from build123d import *

# Parameters (mm, degrees)
BOSS_EXTRUDE1_DEPTH   = 7.62
BOSS_EXTRUDE1_2_DEPTH = 7.62
BOSS_EXTRUDE1_3_DEPTH = 7.62
BOSS_EXTRUDE1_4_DEPTH = 7.62
SKETCH2_W             = 132.9538108
SKETCH2_H             = 20
BOSS_EXTRUDE2_DEPTH   = 6.35
LPATTERN2_COUNT       = 2
LPATTERN2_PITCH       = 75.4126
CUT_EXTRUDE1_DEPTH    = 125.148300392
FILLET1_R             = 2.54
SKETCH6_W             = 25.4
SKETCH6_H             = 25.4
BOSS_EXTRUDE7_DEPTH   = 12.7
FILLET3_R             = 7.62
FILLET5_R             = 7.62
SKETCH11_R            = 1.984375
CUT_EXTRUDE3_DEPTH    = 137.653262418
SKETCH13_R            = 3.5
CUT_EXTRUDE5_DEPTH    = 127.945019246
FILLET6_R             = 2.54


with BuildPart() as part:
    # Sketch1 → Boss-Extrude1 (new body)
    with BuildSketch(Plane(origin=(0, 0, 0), x_dir=(1, 0, 0), z_dir=(0, 1, 0))):
        Polygon((-2.9718, 10), (-2.9718, 7.714), (-4.4450054, 7.714), (-4.4450054, 6.444), (-2.9718, 4.158), (2.9718, 4.158), (4.4449946, 6.444), (4.4449946, 7.714), (2.9718, 7.714), (2.9718, 10), align=None)
    boss_extrude1 = extrude(amount=BOSS_EXTRUDE1_DEPTH)



with BuildPart() as body_2:
    # Sketch1 → Boss-Extrude1 2 (new body)
    with BuildSketch(Plane(origin=(0, 0, 0), x_dir=(1, 0, 0), z_dir=(0, 1, 0))):
        Polygon((4.158, -2.9718), (4.158, 2.9718), (6.444, 4.4449946), (7.714, 4.4449946), (7.714, 2.9718), (10, 2.9718), (10, -2.9718), (7.714, -2.9718), (7.714, -4.4450054), (6.444, -4.4450054), align=None)
    boss_extrude1_2 = extrude(amount=BOSS_EXTRUDE1_2_DEPTH)


with BuildPart() as body_3:
    # Sketch1 → Boss-Extrude1 3 (new body)
    with BuildSketch(Plane(origin=(0, 0, 0), x_dir=(1, 0, 0), z_dir=(0, 1, 0))):
        Polygon((4.4450054, -6.444), (2.9718, -4.158), (-2.9718, -4.158), (-4.4449946, -6.444), (-4.4449946, -7.714), (-2.9718, -7.714), (-2.9718, -10), (2.9718, -10), (2.9718, -7.714), (4.4450054, -7.714), align=None)
    boss_extrude1_3 = extrude(amount=BOSS_EXTRUDE1_3_DEPTH)


with BuildPart() as body_4:
    # Sketch1 → Boss-Extrude1 4 (new body)
    with BuildSketch(Plane(origin=(0, 0, 0), x_dir=(1, 0, 0), z_dir=(0, 1, 0))):
        Polygon((-10, -2.9718), (-10, 2.9718), (-7.714, 2.9718), (-7.714, 4.4450054), (-6.444, 4.4450054), (-4.158, 2.9718), (-4.158, -2.9718), (-6.444, -4.4449946), (-7.714, -4.4449946), (-7.714, -2.9718), align=None)
    boss_extrude1_4 = extrude(amount=BOSS_EXTRUDE1_4_DEPTH)


with BuildPart() as part_1:
    add(part.part)

    add(body_2.part)  # Boss-Extrude2 merges body 2

    add(body_3.part)  # Boss-Extrude2 merges body 3

    add(body_4.part)  # Boss-Extrude2 merges body 4
    # Sketch2 → Boss-Extrude2 (add)
    with BuildSketch(Plane.XZ):
        with Locations((-56.4769054, 0)):
            Rectangle(SKETCH2_W, SKETCH2_H)
    extrude(amount=BOSS_EXTRUDE2_DEPTH)

    # LPattern2: Boss-Extrude1, Boss-Extrude1 2, Boss-Extrude1 3, Boss-Extrude1 4 ×2
    with Locations(*[(-i * LPATTERN2_PITCH, 0, 0) for i in range(1, LPATTERN2_COUNT)]):
        add(boss_extrude1)
        add(boss_extrude1_2)
        add(boss_extrude1_3)
        add(boss_extrude1_4)

    # Sketch4 → Cut-Extrude1 (cut, through all)
    with BuildSketch(Plane(origin=(0, -6.35, 0), x_dir=(-1, 0, 0), z_dir=(0, -1, 0))):
        Polygon((122.9538108, -10), (85.4126108, -10), (122.9538108, -0.2108), align=None)
    extrude(amount=-CUT_EXTRUDE1_DEPTH, mode=Mode.SUBTRACT)

    # Fillet1
    fillet1_edges = [part_1.edges().sort_by_distance(p)[0] for p in [
        (-85.4126108, -3.175, 10),
    ]]
    fillet(fillet1_edges, radius=FILLET1_R)

    # Sketch6 → Boss-Extrude7 (add)
    with BuildSketch(Plane.ZY.offset(122.9538108)):
        with Locations((-12.4892, 6.35)):
            Rectangle(SKETCH6_W, SKETCH6_H)
    extrude(amount=-BOSS_EXTRUDE7_DEPTH)

    # Fillet3
    fillet3_edges = [part_1.edges().sort_by_distance(p)[0] for p in [
        (-110.2538108, 0, -4.8946),
        (-110.2538108, -3.175, -10),
    ]]
    fillet(fillet3_edges, radius=FILLET3_R)

    # Fillet5
    # the kernel refuses this fillet: 7.62 mm, written as the material it takes off along each edge
    with BuildSketch(Plane(origin=(-110.2538108, 38.1, 0.2108), x_dir=(-1, 0, 0), z_dir=(0, -1, 0))) as fillet5_piece_1:
        with BuildLine():
            CenterArc((FILLET5_R, FILLET5_R), FILLET5_R, 180, 90)
            Line((0, FILLET5_R), (0, 0))
            Line((0, 0), (FILLET5_R, 0))
        make_face()
    extrude(amount=30.48, mode=Mode.SUBTRACT)
    with BuildSketch(Plane(origin=(-102.6338108, 7.62, 0.2108), x_dir=(0.5976672776328267, 0.8017442392976488, 0), z_dir=(-0.8017442392976488, 0.5976672776328267, 0))) as fillet5_piece_2_section:
        with BuildLine():
            CenterArc((7.62 + FILLET5_R, FILLET5_R), FILLET5_R, 180, 90)
            Line((7.62, FILLET5_R), (7.62, 0))
            Line((7.62, 0), (7.62 + FILLET5_R, 0))
        make_face()
    fillet5_piece_2 = revolve(axis=Axis((-102.6338108, 7.62, 0.2108), (0, 0, -1)), revolution_arc=233.296989237, mode=Mode.PRIVATE)
    fillet5_piece_2 = split(fillet5_piece_2, bisect_by=Plane(origin=(-108.348345601, 0, -2.163807766), z_dir=(0, 1, 0)), keep=Keep.TOP, mode=Mode.PRIVATE)
    add(fillet5_piece_2, mode=Mode.SUBTRACT)

    # Sketch11 → Cut-Extrude3 (cut, through all)
    with BuildSketch(Plane.ZY.offset(122.9538108)):
        with Locations((-12.4892, 6.35)):
            Circle(SKETCH11_R)
    extrude(amount=-CUT_EXTRUDE3_DEPTH, mode=Mode.SUBTRACT)

    # Sketch13 → Cut-Extrude5 (cut, through all)
    with BuildSketch(Plane(origin=(0, 0, 0), x_dir=(1, 0, 0), z_dir=(0, 1, 0))):
        with Locations(Location((0, 0, 0), (0, 0, 270))):
            Circle(SKETCH13_R)
        with Locations(Location((-75.4126, 0, 0), (0, 0, 270))):
            Circle(SKETCH13_R)
    extrude(amount=-CUT_EXTRUDE5_DEPTH, mode=Mode.SUBTRACT)

    # Fillet6
    fillet6_edges = [part_1.edges().sort_by_distance(p)[0] for p in [
        (0, -6.35, -3.5),
        (-75.4126, -6.35, -3.5),
    ]]
    fillet(fillet6_edges, radius=FILLET6_R)


solid = part_1.part
Geometry check sheet. Reference: the model listing, model coordinates, mm. A direction names the side the tool comes from. Give positions to 0.01 mm unless a question says otherwise; leave off trailing zeros. Write each loop counter-clockwise with the first axis right and the second up, starting at its lowest first coordinate (ties: lowest second). Pieces come first, ordered by that corner, then holes. Notation, with made-up numbers: (62.5, 79.5) - (100.5, 79.5) arc R22 cw to (100.5, 99.5) - close; hole circle Ø10 at (17.25, 76.5). An arc over 180 degrees is marked (long way). Put each result on its own line as item: value.
1. Set-up check for faces 4 (the cylindrical face through (-116.333, 5.59, -10.656)), 5 (the flat face through (-120, 9, 0.211)), 6 (the flat face through (2.972, 4, -9)), 7 (the flat face through (-84, 4, -2.972)), 8 (the flat face through (-79.571, 4, 0)): record each of +Z, -Z, +X, -X, +Y, -Y from which the full face is reachable in a straight line by a thin tool's end or side.
Ans:
face 4: +X, -X
face 5: +Z, -X, +Y
face 6: -Z, +X, +Y
face 7: -Z, +Y
face 8: +Y
2. Sectioned sample at C-C, the plane x = -26.5. Enter the section's corners in (y, z), plus the area to 3 significant figures.
Ans:
outline: (-6.35, -10) - (0, -10) - (0, 10) - (-6.35, 10) - close
area: 127 mm²
3. Sectioned sample at B-B, the plane y = -2.25. Enter the section's corners in (x, z).
Ans:
outline: (-122.95, -25.19) - (-110.25, -25.19) - (-110.25, -17.62) arc R7.62 cw to (-102.63, -10) - (10, -10) - (10, 10) - (-85.09, 10) arc R2.54 ccw to (-85.73, 9.92) - (-122.95, 0.21) - close; hole circle Ø7 at (-75.41, 0); hole circle Ø7 at (0, 0)
4. Sectioned sample at D-D, the plane y = 6.35. Give the number of separate pieces and of enclosed holes in the cut face, plus the area to 3 significant figures.
Ans:
separate pieces: 10
enclosed holes: 0
area: 596 mm²
5. Thickness scan on line 1 (X direction, y = -1.65, z = 0); line 2 (X direction, y = 6.5, z = -5); line 3 (Y direction, x = -26, z = 5). Record the ranges inside material, lowest first.
Ans:
line 1: x = -122.95 to -78.91, -71.91 to -3.5, 3.5 to 10
line 2: x = -122.95 to -110.57, -78.93 to -71.9, -3.51 to 3.51
line 3: y = -6.35 to 0
6. Draft check along Z on faces 1 (the flat face through (0, 4, 4.158)), 2 (the flat face through (-67, 4, 2.972)), 3 (the flat face through (-110.254, 9, -18)). Enter one of: +Z half, -Z half, draft (parallel to the pull), parting line (faces both ways), or undercut.
Ans:
face 1: undercut
face 2: +Z half
face 3: draft
7. Sectioned sample at A-A, the plane x = 0. Enter the section's corners in (y, z), plus the area to 3 significant figures.
Ans:
outline: (-6.35, -10) - (7.62, -10) - (7.62, -4.16) - (0, -4.16) - (0, -3.5) - (-3.81, -3.5) arc R2.54 ccw to (-6.35, -6.04) - close; (-6.35, 6.04) arc R2.54 ccw to (-3.81, 3.5) - (0, 3.5) - (0, 4.16) - (7.62, 4.16) - (7.62, 10) - (-6.35, 10) - close
area: 169 mm²
8. Go/stop test with flat-tipped pins: pin 1 (1.5 mm diameter, centred on x = -42.5, z = -1, fed in from +Y); pin 2 (4.5 mm diameter, centred on x = -0.5, z = -8, fed in from +Y); pin 3 (8 mm diameter, centred on y = 12, z = -20.5, fed in from +X); pin 4 (12 mm diameter, centred on y = 4, z = -12, fed in from +X). Record where each tip stops, or that it passes through.
Ans:
pin 1: stops at y = 0
pin 2: stops at y = 7.62
pin 3: stops at x = -110.25
pin 4: stops at x = 10
